```python
from build123d import *

# Parameters (mm, degrees)
F1_DEPTH = 76.2
F3_DEPTH = 50.8
F5_DEPTH = 25.4


with BuildPart() as f1:
    # F0 (on Front) → F1 (new body)
    with BuildSketch(Plane.XZ):
        Polygon((0, 50.8), (0, 0), (152.4, 0), (152.4, 25.4), (25.4, 25.4), (25.4, 50.8), align=None)
    extrude(amount=-F1_DEPTH)

    # F2 (on Front) → F3 (join)
    with BuildSketch(Plane.XZ):
        Polygon((25.018999, 50.418999), (25.018999, 25.273001), (152.018994, 25.273001), align=None)
    extrude(amount=-F3_DEPTH)

    # F4 (on Front) → F5 (cut)
    with BuildSketch(Plane.XZ):
        Polygon((152.272999, 25.273001), (25.527, 51.181), (25.527, 25.273001), (28.067, 25.273001), align=None)
    extrude(amount=-F5_DEPTH, mode=Mode.SUBTRACT)


solid = f1.part
```
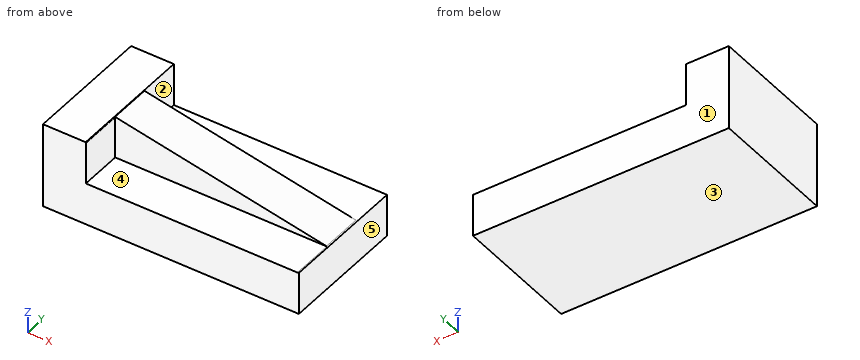
Read the model definition and answer for the solid it produces. Units are mm, in the model's axes. Face numbers are marked on the shaded views. A direction names the side the tool comes from. Coordinates: 2 decimals unless noted, no trailing zeros. Write each loop counter-clockwise with the first axis right and the second up, starting at its lowest first coordinate (ties: lowest second). Pieces come first, ordered by that corner, then holes. Notation, with made-up numbers: (45, 47.5) -> (77, 47.5) arc R19 ccw to (77, 60.5) -> close; hole circle Ø2 at (30, -20.75). An arc over 180 degrees is marked (long way). Return JSON: item names as keys, results as strings.
1. Determine the mould class of the marked faces 3, 4 and 5 for opening direction X: pulls with the +X half, pulls with the -X half, needs draft (parallel to the pull), parting line crosses it, or undercut.
Found:
{"face 3": "needs draft", "face 4": "undercut", "face 5": "pulls with the +X half"}
2. Each of these flat-tipped pins is pushed along its axis until it touches: P1, Ø8, axis at x = 100, y = 26.5, coming from the -Z side; P2, Ø12.5, axis at x = 60.5, z = 41.5, coming from the +Y side; P3, Ø7.5, axis at x = 73, z = 34.5, coming from the -Y side; P4, Ø2, axis at y = 9, z = 36.5, coming from the +X side. Where does it stop, or does it pass through?
Found:
{"P1": "z = 0", "P2": "y = 50.8", "P3": "y = 25.4", "P4": "x = 25.53"}
3. A cutting plane is placed at A-A (y = 7.5). Determine the outline of the cut face in (x, z), and give its area (3 significant figures).
Found:
{"outline": "(0, 0) -> (152.4, 0) -> (152.4, 25.4) -> (151.65, 25.4) -> (152.27, 25.27) -> (25.53, 25.27) -> (25.53, 50.32) -> (25.4, 50.34) -> (25.4, 50.8) -> (0, 50.8) -> close", "area": "4,500 mm2"}
4. A cutting plane is placed at B-B (x = 73.5). Determine the outline of the cut face in (y, z).
Found:
{"outline": "(0, 0) -> (76.2, 0) -> (76.2, 25.4) -> (50.8, 25.4) -> (50.8, 40.82) -> (25.4, 40.82) -> (25.4, 25.27) -> (0, 25.27) -> close"}
5. Find the intervals of material crossed by line 1 along Y through (x, z) = (129.5, 29); line 2 along Z through (x, y) = (47, 14); line 3 along X through (y, z) = (56, 40.5), in increasing order. Write a range as from..to.
Found:
{"line 1": "25.4..50.8", "line 2": "0..25.27", "line 3": "0..25.4"}
6. A cutting plane is placed at D-D (y = 38). Determine the outline of the cut face in (x, z), and give its area (3 significant figures).
Found:
{"outline": "(0, 0) -> (152.4, 0) -> (152.4, 25.4) -> (151.38, 25.4) -> (25.4, 50.34) -> (25.4, 50.8) -> (0, 50.8) -> close", "area": "6,090 mm2"}
7. A cutting plane is placed at C-C (z = 43). Determine the outline of the cut face in (x, y), and give its area (3 significant figures).
Found:
{"outline": "(0, 0) -> (25.53, 0) -> (25.53, 25.4) -> (62.49, 25.4) -> (62.49, 50.8) -> (25.4, 50.8) -> (25.4, 76.2) -> (0, 76.2) -> close", "area": "2,880 mm2"}
8. A tool of negligible diameter and unlimited length cuts with its end or side. For the marked faces 1 and 2, from which of +Z, -Z, +X, -X, +Y, -Y can it reach the whole face along a straight path? Write none if from no direction.
Found:
{"face 1": "+Z, -Z, +X, -X, +Y", "face 2": "+Z, +X, +Y"}
